```python
from build123d import *

# Parameters (mm, degrees)
F0_R           = 25.4061794045
F1_DEPTH       = 25.4
F2_D           = 5.5
F2_CBORE_D     = 9.75
F2_CBORE_DEPTH = 5


with BuildPart() as f1:
    # F0 (on Front) → F1 (new body)
    with BuildSketch(Plane.XZ):
        Circle(F0_R)
    extrude(amount=F1_DEPTH)

    # F2 (through all)
    with Locations(Plane(origin=(0, 0, 0), x_dir=(1, 0, 0), z_dir=(0, 1, 0))):
        with Locations((0, -18.4791404754), (-13.0667255406, -13.0667255406), (-18.4791404754, 0), (-13.0667255406, 13.0667255406), (0, 18.4791404754), (13.0667255406, 13.0667255406), (18.4791404754, 0), (13.0667255406, -13.0667255406)):
            CounterBoreHole(F2_D / 2, F2_CBORE_D / 2, F2_CBORE_DEPTH)


solid = f1.part
```
Build history of the part. All positions in model axes, mm. A direction names the side the tool comes from. Coordinates: 2 decimals unless noted, no trailing zeros. Order: outer loops, then holes, each group sorted by start corner. A loop starts at its lowest first (then second) coordinate and runs counter-clockwise, first axis right, second up. Notation, with made-up numbers: (19, -37) -> (44, -37) arc R21 ccw to (44, -14) -> close; hole circle Ø10 at (58, -13.5). An arc over 180 degrees is marked (long way). Answer in a Markdown table with one row per item. Add a question column.
Q1. Mould opens along X. For faces 3 (the face through (2, -5, 21)), 4 (the face through (-20.16, -12.52, -15.46)), 5 (the face through (0, -25.4, 0)) say: +X half, -X half, draft (parallel to the pull), parting line (faces both ways), or undercut.
Q2. Wall check: line 1 along Z through (x, y) = (0, -1.05); line 2 along Z through (x, y) = (11, -15.5); line 3 along Z through (x, y) = (14, -1.25). Give the ranges that are in metal, low to high. Write a range as [from, to].
Q3. Drop flat-ended pins along their axis: pin 1 (7 mm diameter, centred on x = -13.07, z = 13.07, fed in from +Y); pin 2 (1 mm diameter, centred on x = -20, z = -17.5, fed in from +Y); pin 3 (10 mm diameter, centred on y = -7, z = 16.5, fed in from +X); pin 4 (8 mm diameter, centred on x = -12.5, y = -21, fed in from +Z). Give the stop position or say it passes through.
Q4. Which spindle directions (+Z, -Z, +X, -X, +Y, -Y) get a long thin tool onto all of the face, cutting with end or side? Do faces 1 (the face through (0, 0, 0)), 2 (the face through (-1.057, -2.465, 23.238)). Say none if no direction does.
Q5. Band-saw the part on C-C, the plane x = 20.5. List the corners of the cut face in (y, z), then the cut area to 3 significant figures.
Q6. Band-saw the part on A-A, the plane x = 0. List the corners of the cut face in (y, z), then the cut area to 3 significant figures.
Q7. Band-saw the part on B-B, the plane z = 0. List the corners of the cut face in (x, y).
Q8. Band-saw the part on D-D, the plane y = -6. Give the number of separate pieces and of enclosed holes in the cut face, then the cut area to 3 significant figures.
Answers follow:
| question | item | result |
|---|---|---|
| 1 | face 3 | undercut |
| 1 | face 4 | parting line |
| 1 | face 5 | draft |
| 2 | line 1 | [-25.41, -23.35], [-13.6, 13.6], [23.35, 25.41] |
| 2 | line 2 | [-22.9, -14.88], [-11.25, 11.25], [14.88, 22.9] |
| 2 | line 3 | [-21.2, -17.85], [-8.28, -1.92], [1.92, 8.28], [17.85, 21.2] |
| 3 | pin 1 | y = -5 |
| 3 | pin 2 | through |
| 3 | pin 3 | x = 22.65 |
| 3 | pin 4 | z = 23.94 |
| 4 | face 1 | +Z, -Z, +X, -X, +Y |
| 4 | face 2 | +Y |
| 5 | outline | (-25.4, -15.01) -> (0, -15.01) -> (0, -4.44) -> (-5, -4.44) -> (-5, -1.87) -> (-25.4, -1.87) -> close; (-25.4, 1.87) -> (-5, 1.87) -> (-5, 4.44) -> (0, 4.44) -> (0, 15.01) -> (-25.4, 15.01) -> close |
| 5 | area | 642 mm^2 |
| 6 | outline | (-25.4, -25.41) -> (0, -25.41) -> (0, -23.35) -> (-5, -23.35) -> (-5, -21.23) -> (-25.4, -21.23) -> close; (-25.4, -15.73) -> (-5, -15.73) -> (-5, -13.6) -> (0, -13.6) -> (0, 13.6) -> (-5, 13.6) -> (-5, 15.73) -> (-25.4, 15.73) -> close; (-25.4, 21.23) -> (-5, 21.23) -> (-5, 23.35) -> (0, 23.35) -> (0, 25.41) -> (-25.4, 25.41) -> close |
| 6 | area | 969 mm^2 |
| 7 | outline | (-25.41, -25.4) -> (-21.23, -25.4) -> (-21.23, -5) -> (-23.35, -5) -> (-23.35, 0) -> (-25.41, 0) -> close; (-15.73, -25.4) -> (15.73, -25.4) -> (15.73, -5) -> (13.6, -5) -> (13.6, 0) -> (-13.6, 0) -> (-13.6, -5) -> (-15.73, -5) -> close; (21.23, -25.4) -> (25.41, -25.4) -> (25.41, 0) -> (23.35, 0) -> (23.35, -5) -> (21.23, -5) -> close |
| 8 | separate pieces | 1 |
| 8 | enclosed holes | 8 |
| 8 | area | 1,840 mm^2 |
